from build123d import *

# Parameters (mm, degrees)
POWIERZCHNIA_PO_CZ2_START   = -125
POWIERZCHNIA_PO_CZ2_DEPTH   = 125
POWIERZCHNIA_PO_CZ2_START_2 = -27
POWIERZCHNIA_PO_CZ2_2_DEPTH = 54
SZKIC4_R                    = 18
WYTNIJ_WYCI_GNI_CIE1_DEPTH  = 625.830377118


with BuildPart() as part:
    # Powierzchnia-Połącz2: read off the stored shape, not the designer's step
    # Powierzchnia-Połącz2 outline → Powierzchnia-Połącz2 (new body)
    with BuildSketch(Plane.YZ.offset(POWIERZCHNIA_PO_CZ2_START)):
        with BuildLine():
            add(Edge.make_bspline(
                [(-27, -125), (-27, -65.312641889), (-22.885580179, -22.821723351), (-17.654979183, 3.50737937)],
                knots=[0, 0, 0, 0, 1, 1, 1, 1], degree=3))
            Line((-27, -125), (-27, -572))
            Line((-27, -572), (27, -572))
            Line((27, -572), (27, -125))
            add(Edge.make_bspline(
                [(17.654979183, 3.50737937), (22.885580179, -22.821723351), (27, -65.312641889), (27, -125)],
                knots=[0, 0, 0, 0, 1, 1, 1, 1], degree=3))
            ThreePointArc((17.654979183, 3.50737937), (0, 18), (-17.654979183, 3.50737937))
        make_face()
    extrude(amount=POWIERZCHNIA_PO_CZ2_DEPTH)

    # Powierzchnia-Po_cz2 2 outline → Powierzchnia-Po_cz2 2 (cut)
    with BuildSketch(Plane(origin=(0, 0, 0), x_dir=(1, 0, 0), z_dir=(0, 1, 0)).offset(POWIERZCHNIA_PO_CZ2_START_2)):
        with BuildLine():
            Line((-70, 55), (-70, -20))
            Line((-70, -20), (0, -20))
            Line((0, -20), (0, 125))
            ThreePointArc((0, 125), (-49.497474683, 104.497474683), (-70, 55))
        make_face()
        with BuildLine():
            ThreePointArc((-97, 283), (-68.589357775, 214.410642225), (0, 186))
            Line((0, 186), (0, 572))
            Line((0, 572), (-97, 572))
            Line((-97, 572), (-97, 283))
        make_face()
    extrude(amount=POWIERZCHNIA_PO_CZ2_2_DEPTH, mode=Mode.SUBTRACT)

    # Lustro1: part across plane


with BuildPart() as part_1:
    add(part.part)
    add(part.part.mirror(Plane(origin=(0, 0, 0), x_dir=(0, 0, 1), z_dir=(1, 0, 0))))

    # Szkic4 → Wytnij-wyciągnięcie1 (cut, through all)
    with BuildSketch(Plane(origin=(-125, 0, 0), x_dir=(0, 0, -1), z_dir=(1, 0, 0))):
        Circle(SZKIC4_R)
    extrude(amount=WYTNIJ_WYCI_GNI_CIE1_DEPTH, mode=Mode.SUBTRACT)


solid = part_1.part
Model file for the job. Use its own axes, mm. A direction names the side the tool comes from. Coordinates: 2 decimals unless noted, no trailing zeros. Order: outer loops, then holes, each group sorted by start corner. A loop starts at its lowest first (then second) coordinate and runs counter-clockwise, first axis right, second up. Notation, with made-up numbers: (83, 27.25) -> (136, 27.25) arc R24 ccw to (136, 56.25) -> close; hole circle Ø11 at (-37.75, -5). An arc over 180 degrees is marked (long way). Return JSON: item names as keys, results as strings. Group by question number.
Item 1: Saw through at A-A on z = -352.5. Write the cut outline in (x, y), then the cut area to 3 significant figures.
Item 2: Wall check: line 1 along X through (y, z) = (9.5, -44.5); line 2 along X through (y, z) = (2.5, -319); line 3 along Y through (x, z) = (98, 0). Give the ranges that are in metal, low to high. Write a range as [from, to].
Item 3: Pull direction Z, two halves, no side cores. Call faces 1 (the cylindrical face through (-98, 0, -18)), 2 (the flat face through (111, 0, -572)), 3 (the flat face through (-97, 0, -430)): pulls with the +Z half, pulls with the -Z half, needs draft (parallel to the pull), parting line crosses it, or undercut.
Item 4: Tool access for faces 4 (the cylindrical face through (97, 0, -18)), 5 (the flat face through (-70, 0, -33)), 6 (the flat face through (97, 0, -430)): list every direction of +Z, -Z, +X, -X, +Y, -Y with a clear straight run to the whole face (end or side of a thin tool).
Item 5: Flat gauge pins, fed straight in: P1, Ø6, axis at x = 22.5, y = 19, coming from the +Z side; P2, Ø6, axis at x = -77, y = 19.5, coming from the -Z side; P3, Ø10, axis at x = 59, y = -20.5, coming from the +Z side. Where does each tip first touch, or does it go through?
Item 6: Saw through at B-B on y = 0. Write the cut outline in (x, z).
Values found:
{
 "1": {"outline": "(-125, -27) -> (-97, -27) -> (-97, 27) -> (-125, 27) -> close; (97, -27) -> (125, -27) -> (125, 27) -> (97, 27) -> close", "area": "3,020 mm2"},
 "2": {"line 1": "x = [-125, -70], [70, 125]", "line 2": "x = [-125, -97], [97, 125]", "line 3": "y = [-18.33, -18], [18, 18.33]"},
 "3": {"face 1": "undercut", "face 2": "pulls with the -Z half", "face 3": "needs draft"},
 "4": {"face 4": "+X, -X", "face 5": "+Z, +Y, -Y", "face 6": "-Z, +Y, -Y"},
 "5": {"P1": "stops at z = -120.19", "P2": "stops at z = -228.15", "P3": "stops at z = -83.35"},
 "6": {"outline": "(-125, -572) -> (-97, -572) -> (-97, -283) arc R97 cw to (97, -283) -> (97, -572) -> (125, -572) -> (125, -18) -> (70, -18) -> (70, -55) arc R70 cw to (-70, -55) -> (-70, -18) -> (-125, -18) -> close"}
}
